Could you check a few things on this model? Use its own coordinates, in mm. A direction names the side the tool comes from. Coordinates: 2 decimals unless noted, no trailing zeros. Loops run counter-clockwise (first coordinate to the right, second up) from the corner with the lowest first, then second, coordinate; pieces in that order, holes last.
1) Will these pins go through, and if not, where does the flat tip stop? P1, Ø9, axis at x = 27.5, y = 5, coming from the +Z side; P2, Ø5, axis at y = -6.5, z = 15.5, coming from the +X side; P3, Ø1, axis at x = 6, z = 18, coming from the +Y side.
2) For faces 1 (the face through (6, 1.502, 13)), 2 (the face through (12, 0, 0)), which set-ups out of +Z, -Z, +X, -X, +Y, -Y let a thin tool reach every point of the face, with its end or its side?
3) Imagine slicing it at C-C on z = 10.5. Please give me the cut outline in (x, y).
4) Imagine slicing it at B-B on z = 15.5. Please give me the cut outline in (x, y).
5) Thinking about a two-plate mould opening in X: for faces 3 (the face through (7.2, 0, 13)), 4 (the face through (25, 0, 12.7)), 5 (the face through (16.77, -12.94, 6.26)), which applies, released by +X, released by -X, zero draft, split by the parting line, or undercut?
6) If I drill on line 1 along Z through (x, y) = (29, -8.5); line 2 along X through (y, z) = (-4, 21.75), over which ranges is the centre line in solid material (lowest first)?
7) Imagine slicing it at A-A on x = 29. Please give me the cut outline in (y, z), plus the area to 3 significant figures.
```python
from build123d import *

# Parameters (mm, degrees)
F0_R     = 4.061318
F1_DEPTH = 12.7
F2_DEPTH = 25.4
F3_R     = 1.22642


with BuildPart() as f1:
    # F0 (on Top) → F1 (new body)
    with BuildSketch(Plane.XY):
        with BuildLine():
            ThreePointArc((2.511697, 15.282841), (11.806241, 10.024297), (15.487861, 0))
            ThreePointArc((15.487861, 0), (11.806241, -10.024297), (2.511697, -15.282841))
            Line((2.511697, -15.282841), (31.435615, -10.529267))
            ThreePointArc((31.435615, -10.529267), (40.375675, 0), (31.435615, 10.529267))
            Line((31.435615, 10.529267), (2.511697, 15.282841))
        make_face()
        with Locations((31.435615, 0)):
            Circle(F0_R, mode=Mode.SUBTRACT)
        with BuildLine():
            ThreePointArc((2.511697, -15.282841), (11.806241, -10.024297), (15.487861, 0))
            ThreePointArc((15.487861, 0), (11.806241, 10.024297), (2.511697, 15.282841))
            ThreePointArc((2.511697, 15.282841), (-15.487861, 0), (2.511697, -15.282841))
        make_face()
        with BuildLine():
            ThreePointArc((-5.276986, 1.502324), (0, 5.486671), (5.276986, 1.502324))
            Line((5.276986, 1.502324), (7.19986, 1.502324))
            Line((7.19986, 1.502324), (7.19986, -1.577626))
            Line((7.19986, -1.577626), (5.254965, -1.577626))
            ThreePointArc((5.254965, -1.577626), (0, -5.486671), (-5.254965, -1.577626))
            Line((-5.254965, -1.577626), (-7.429904, -1.577626))
            Line((-7.429904, -1.577626), (-7.429904, 1.502324))
            Line((-7.429904, 1.502324), (-5.276986, 1.502324))
        make_face(mode=Mode.SUBTRACT)
        with BuildLine():
            ThreePointArc((-5.254965, -1.577626), (-5.486531, -0.039228), (-5.276986, 1.502324))
            Line((-5.276986, 1.502324), (-7.429904, 1.502324))
            Line((-7.429904, 1.502324), (-7.429904, -1.577626))
            Line((-7.429904, -1.577626), (-5.254965, -1.577626))
        make_face()
    extrude(amount=F1_DEPTH)

    # F0 (on Top) → F2 (join)
    with BuildSketch(Plane.XY):
        with BuildLine():
            ThreePointArc((2.511697, -15.282841), (11.806241, -10.024297), (15.487861, 0))
            ThreePointArc((15.487861, 0), (11.806241, 10.024297), (2.511697, 15.282841))
            ThreePointArc((2.511697, 15.282841), (-15.487861, 0), (2.511697, -15.282841))
        make_face()
        with BuildLine():
            ThreePointArc((-5.276986, 1.502324), (0, 5.486671), (5.276986, 1.502324))
            Line((5.276986, 1.502324), (7.19986, 1.502324))
            Line((7.19986, 1.502324), (7.19986, -1.577626))
            Line((7.19986, -1.577626), (5.254965, -1.577626))
            ThreePointArc((5.254965, -1.577626), (0, -5.486671), (-5.254965, -1.577626))
            Line((-5.254965, -1.577626), (-7.429904, -1.577626))
            Line((-7.429904, -1.577626), (-7.429904, 1.502324))
            Line((-7.429904, 1.502324), (-5.276986, 1.502324))
        make_face(mode=Mode.SUBTRACT)
        with BuildLine():
            ThreePointArc((-5.254965, -1.577626), (-5.486531, -0.039228), (-5.276986, 1.502324))
            Line((-5.276986, 1.502324), (-7.429904, 1.502324))
            Line((-7.429904, 1.502324), (-7.429904, -1.577626))
            Line((-7.429904, -1.577626), (-5.254965, -1.577626))
        make_face()
    extrude(amount=F2_DEPTH)

    # F3
    f3_edges = [f1.edges().sort_by_distance(p)[0] for p in [
        (-2.511697, 15.282841, 25.4),
    ]]
    fillet(f3_edges, radius=F3_R)


solid = f1.part
```
Filled in:
1. P1: stops at z = 12.7
1. P2: stops at x = 14.96
1. P3: stops at y = 14.48
2. face 1: +Z, -Z
2. face 2: -Z, +X, -X, +Y, -Y
3. outline: (2.51, -15.28) - (31.44, -10.53) arc R10.67 ccw to (31.44, 10.53) - (2.51, 15.28) arc R15.49 ccw (long way) to start; hole (-5.28, 1.5) arc R5.49 ccw to (-5.25, -1.58) arc R5.49 ccw to (5.25, -1.58) - (7.2, -1.58) - (7.2, 1.5) - (5.28, 1.5) arc R5.49 ccw to start; hole circle Ø8.12 at (31.44, 0)
4. outline: (2.51, -15.28) arc R15.49 ccw to (15.49, 0) arc R15.49 ccw to (2.51, 15.28) arc R15.49 ccw (long way) to start; hole (-5.28, 1.5) arc R5.49 ccw to (-5.25, -1.58) arc R5.49 ccw to (5.25, -1.58) - (7.2, -1.58) - (7.2, 1.5) - (5.28, 1.5) arc R5.49 ccw to start
5. face 3: undercut
5. face 4: zero draft
5. face 5: released by +X
6. line 1: z = 0 to 12.7
6. line 2: x = -14.96 to -3.76, 3.76 to 14.96
7. outline: (-10.93, 0) - (-3.25, 0) - (-3.25, 12.7) - (-10.93, 12.7) - close; (3.25, 0) - (10.93, 0) - (10.93, 12.7) - (3.25, 12.7) - close
7. area: 195 mm2
